The listing builds one solid part. Answer for the finished solid, in the listing's coordinates (mm). Face numbers are marked on the shaded views. Coordinates: 2 decimals unless noted, no trailing zeros. Loops run counter-clockwise (first coordinate to the right, second up) from the corner with the lowest first, then second, coordinate; pieces in that order, holes last. Notation, with made-up numbers: M -38.75,24 L -33.75,24 A16 ccw -33.75,41 Z; hole C -21.75,46 d8. An arc over 180 degrees is marked long. Answer in a Markdown table with one row per item. Add a question column.
from build123d import *

# Parameters (mm, degrees)
F0_R     = 12.5
F0_R_2   = 7.5
F1_DEPTH = 25


with BuildPart() as f1:
    # F0 (on Top) → F1 (new body)
    with BuildSketch(Plane.XY):
        with BuildLine():
            ThreePointArc((60.859742, 61.362541), (-0.829779, 84.343763), (-65.360229, 71.322454))
            ThreePointArc((-65.360229, 71.322454), (-68.102494, 69.860047), (-70.805967, 68.327115))
            ThreePointArc((-70.805967, 68.327115), (-72.798151, 29.458795), (-34.389511, 35.743021))
            ThreePointArc((-34.389511, 35.743021), (2.341937, 46.39821), (40.298576, 41.705039))
            ThreePointArc((40.298576, 41.705039), (64.237658, 37.247404), (60.859742, 61.362541))
        make_face()
        with Locations((-56.12801, 48.089586)):
            Circle(F0_R, mode=Mode.SUBTRACT)
        with Locations((53.87199, 48.089586)):
            Circle(F0_R_2, mode=Mode.SUBTRACT)
    extrude(amount=F1_DEPTH)


solid = f1.part
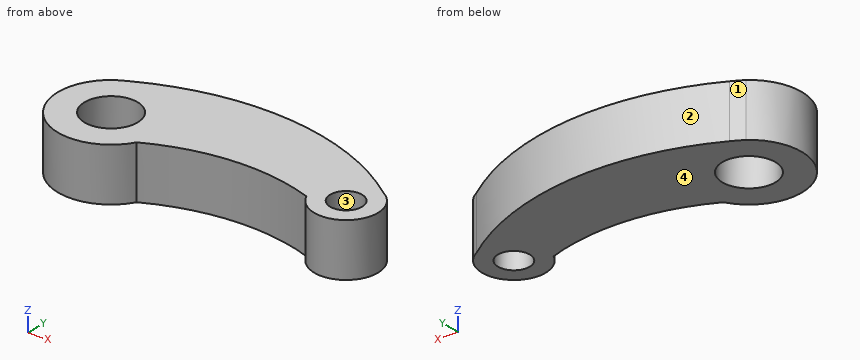
(1) A cutting plane is placed at B-B (y = 57). Give the vertices of the cut face in (x, z), plus the area to 3 significant figures.
(2) Straight lines are drawn through the part: line 1 (X direction, y = 48, z = 8.75); line 2 (X direction, y = 54, z = 14); line 3 (Y direction, x = -46.5, z = 23.5). For each, find the intervals that lie inside material, in ascending order.
(3) A cutting plane is placed at A-A (x = -56). Give the vertices of the cut face in (y, z).
(4) The mould has two halves that part along X. Classify the marked faces 1, 2, 3 and 4: released by +X, released by -X, zero draft, split by the parting line, or undercut.
(5) A cutting plane is placed at D-D (x = 2). Give the vertices of the cut face in (y, z).
(6) A cutting plane is placed at C-C (z = 17.5). Give the vertices of the cut face in (x, y), plus the area to 3 significant figures.
(7) Each of these flat-tipped pins is pushed along its axis until it touches: pin 1 (12 mm diameter, centred on x = -36, z = 7.5, fed in from +Y); pin 2 (1 mm diameter, centred on x = -39.5, z = 22.5, fed in from +Y); pin 3 (10 mm diameter, centred on y = 46, z = 19.5, fed in from -X). Where does it stop, or does it pass through?
Solved:
| question | item | result |
|---|---|---|
| 1 | outline | M -79.49,0 L -64.89,0 L -64.89,25 L -79.49,25 Z; M -47.36,0 L 65.94,0 L 65.94,25 L -47.36,25 Z |
| 1 | area | 3,200 mm² |
| 2 | line 1 | x = -81.13 to -68.63, -43.63 to 46.37, 61.37 to 68.87 |
| 2 | line 2 | x = -80.42 to -67.14, -45.11 to 49.25, 58.49 to 67.66 |
| 2 | line 3 | y = 25.02 to 40.12, 56.06 to 79.12 |
| 3 | outline | M 23.09,0 L 35.59,0 L 35.59,25 L 23.09,25 Z; M 60.59,0 L 75.66,0 L 75.66,25 L 60.59,25 Z |
| 4 | face 1 | released by -X |
| 4 | face 2 | split by the parting line |
| 4 | face 3 | undercut |
| 4 | face 4 | zero draft |
| 5 | outline | M 46.37,0 L 84.09,0 L 84.09,25 L 46.37,25 Z |
| 6 | outline | M -70.81,68.33 A25 ccw long -34.39,35.74 A95 cw 40.3,41.71 A15 ccw long 60.86,61.36 A120 ccw -65.36,71.32 A120 ccw Z; hole C -56.13,48.09 d25; hole C 53.87,48.09 d15 |
| 6 | area | 5,140 mm² |
| 7 | pin 1 | stops at y = 83.08 |
| 7 | pin 2 | stops at y = 81.23 |
| 7 | pin 3 | stops at x = -81.13 |
